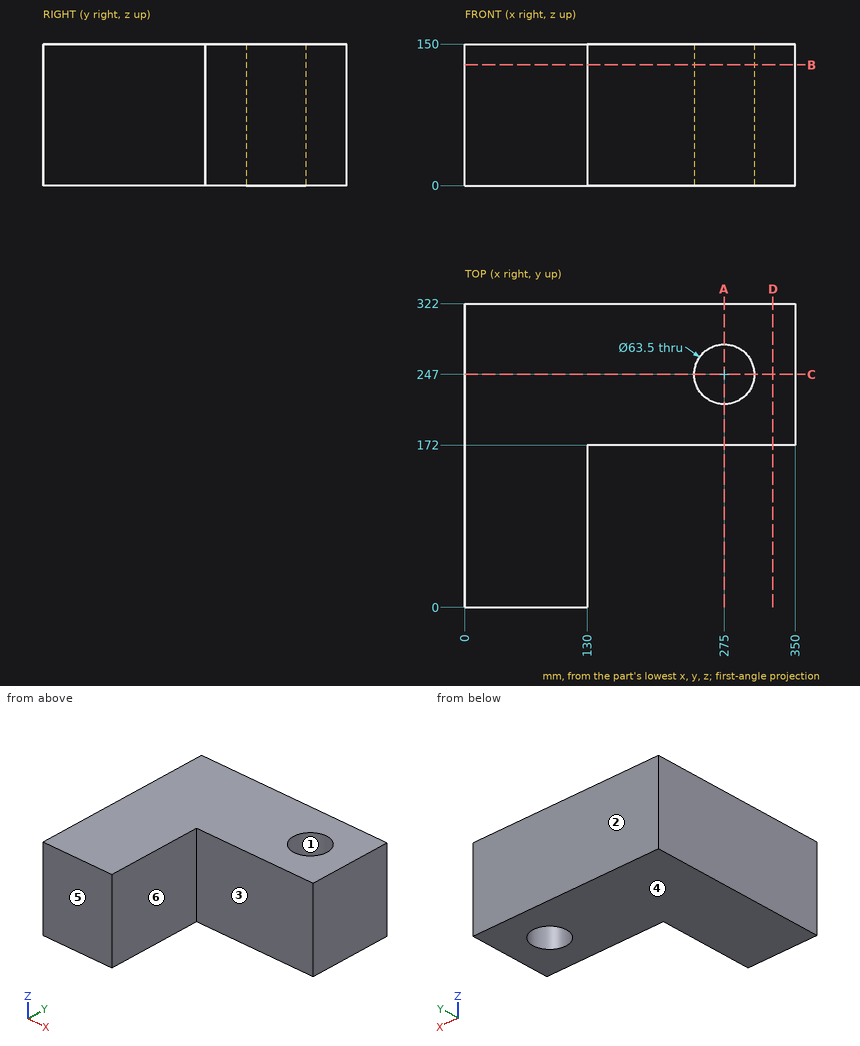
Drawing for the job (mm, zero at the part's lowest x, y, z). A direction names the side the tool comes from. Give positions to 0.01 mm unless a question says otherwise; leave off trailing zeros. Order: outer loops, then holes, each group sorted by start corner. A loop starts at its lowest first (then second) coordinate and runs counter-clockwise, first axis right, second up. Notation, with made-up numbers: (46, -12) - (100, -12) arc R17 cw to (100, 3) - close; hole circle Ø6 at (16.25, 16.25). An arc over 180 degrees is marked (long way). Write item = value, one per line. Start each with the question number.
1. Cut at B-B, the plane z = 128. List the corners of the cut face in (x, y), and give its area (3 significant figures).
2. Cut at C-C, the plane y = 247. List the corners of the cut face in (x, z).
3. Drop flat-ended pins along their axis: P1, Ø3, axis at y = 169, z = 97.5, coming from the +X side; P2, Ø5, axis at y = 273, z = 39.5, coming from the -X side; P3, Ø1.5, axis at x = 207.5, z = 98, coming from the -Y side. Give the stop position or say it passes through.
4. Probe line 1 along X through (y, z) = (247, 103); line 2 along Y through (x, z) = (275, 119); line 3 along X through (y, z) = (23, 87). List the from-to ranges inside material, lowest first.
5. Cut at A-A, the plane x = 275. List the corners of the cut face in (y, z), and give its area (3 significant figures).
6. Two-plate mould, pull along Y, no slides. Class the marked faces 1, 2, 3 and 4: pulls with the +Y half, pulls with the -Y half, needs draft (parallel to the pull), parting line crosses it, or undercut.
7. Which spindle directions (+Z, -Z, +X, -X, +Y, -Y) get a long thin tool onto all of the face, cutting with end or side? Do the marked faces 5 and 6. Say none if no direction does.
8. Cut at D-D, the plane x = 326.5. List the corners of the cut face in (y, z).
Taken from the geometry:
q1.outline = (0, 0) - (130, 0) - (130, 172) - (350, 172) - (350, 322) - (0, 322) - close; hole circle Ø63.5 at (275, 247)
q1.area = 71,700 mm²
q2.outline = (0, 0) - (243.25, 0) - (243.25, 150) - (0, 150) - close; (306.75, 0) - (350, 0) - (350, 150) - (306.75, 150) - close
q3.P1 = 130
q3.P2 = 0
q3.P3 = 172
q4.line_1 = 0 to 243.25, 306.75 to 350
q4.line_2 = 172 to 215.25, 278.75 to 322
q4.line_3 = 0 to 130
q5.outline = (172, 0) - (215.25, 0) - (215.25, 150) - (172, 150) - close; (278.75, 0) - (322, 0) - (322, 150) - (278.75, 150) - close
q5.area = 13,000 mm²
q6.face_1 = undercut
q6.face_2 = pulls with the +Y half
q6.face_3 = pulls with the -Y half
q6.face_4 = needs draft
q7.face_5 = +Z, -Z, +X, -X, -Y
q7.face_6 = +Z, -Z, +X, -Y
q8.outline = (172, 0) - (322, 0) - (322, 150) - (172, 150) - close
